from build123d import *

# Parameters (mm, degrees)
ESBO_O1_W                = 22
ESBO_O1_H                = 36
RESSALTO_EXTRUS_O1_DEPTH = 250
CASCA1_T                 = -2
ESBO_O2_R                = 5
CORTE_EXTRUS_O1_DEPTH    = 10
ESBO_O3_R                = 2.75
CORTE_EXTRUS_O2_DEPTH    = 29


with BuildPart() as part:
    # Esboço1 → Ressalto-extrusão1 (new body)
    with BuildSketch(Plane.XY):
        with Locations((0, 18)):
            Rectangle(ESBO_O1_W, ESBO_O1_H)
    extrude(amount=RESSALTO_EXTRUS_O1_DEPTH)

    # Casca1
    casca1_openings = [part.faces().sort_by_distance(p)[0] for p in [
        (0, 18, 0),
    ]]
    offset(amount=CASCA1_T, openings=casca1_openings, kind=Kind.INTERSECTION)

    # Esboço2 → Corte-extrusão1 (cut)
    with BuildSketch(Plane(origin=(0, 0, 0), x_dir=(-1, 0, 0), z_dir=(0, -1, 0))):
        with Locations(Location((0, -20, 0), (0, 0, 90))):
            Circle(ESBO_O2_R)
        with Locations(Location((0, -40, 0), (0, 0, 90))):
            Circle(ESBO_O2_R)
        with Locations(Location((0, -60, 0), (0, 0, 90))):
            Circle(ESBO_O2_R)
        with Locations(Location((0, -80, 0), (0, 0, 90))):
            Circle(ESBO_O2_R)
        with Locations(Location((0, -100, 0), (0, 0, 90))):
            Circle(ESBO_O2_R)
    extrude(amount=-CORTE_EXTRUS_O1_DEPTH, mode=Mode.SUBTRACT)

    # Esboço3 → Corte-extrusão2 (cut)
    with BuildSketch(Plane(origin=(11, 0, 0), x_dir=(0, 0, -1), z_dir=(1, 0, 0))):
        with Locations(Location((-230, 18, 0), (0, 0, 90))):
            Circle(ESBO_O3_R)
    extrude(amount=-CORTE_EXTRUS_O2_DEPTH, mode=Mode.SUBTRACT)


solid = part.part
Here's how the part is built. I have some questions about the finished solid (model axes, mm). A direction names the side the tool comes from. Coordinates: 2 decimals unless noted, no trailing zeros. Order: outer loops, then holes, each group sorted by start corner. A loop starts at its lowest first (then second) coordinate and runs counter-clockwise, first axis right, second up. Notation, with made-up numbers: (83.5, 49) - (123.5, 49) arc R20 ccw to (123.5, 63) - close; hole circle Ø10 at (-9, 89). An arc over 180 degrees is marked (long way). Use CSV: the item, a comma, the result in double quotes. Start each with the question number.
1. Suppose I cut it at A-A on z = 230. List the corners of the cut face in (x, y) for me, then the cut area to 3 significant figures.
2. For faces 5 (the face through (0, 1, 65)), 6 (the face through (0, 2, 122)), 7 (the face through (10.014, 17.404, 227.315)), which set-ups out of +Z, -Z, +X, -X, +Y, -Y let a thin tool reach every point of the face, with its end or its side?
3. Please list where these lines run through material, in increasing order: line 1 (X direction, y = 17.5, z = 140.5); line 2 (Z direction, x = -9.7, y = 18); line 3 (X direction, y = 0.6, z = 100). Write a range as from..to.
4. I'm going to push flat-ended pins straight in: pin 1 (9 mm diameter, centred on x = 0, z = 80, fed in from -Y); pin 2 (1 mm diameter, centred on x = -4, y = 26.5, fed in from -Z). Where does each tip first touch, or does it pass through?
5. Suppose I cut it at C-C on z = 116.5. List the corners of the cut face in (x, y) for me.
6. Suppose I cut it at B-B on y = 18. List the corners of the cut face in (x, z) for me.
7. If we mould it in two halves opening along Y, with no side actions, what happens to faces 1 (the face through (0, 36, 123)), 2 (the face through (0, 34, 122)), 3 (the face through (0, 18, 248)), 4 (the face through (-1.915, 0.986, 75.381))? For each: +Y half, -Y half, draft (parallel to the pull), parting line (faces both ways), or undercut.
8. Suppose I cut it at D-D on x = 0. List the corners of the cut face in (y, z) for me, then the cut area to 3 significant figures.
Output:
1,outline,"(-11, 0) - (11, 0) - (11, 15.25) - (9, 15.25) - (9, 2) - (-9, 2) - (-9, 15.25) - (-11, 15.25) - close; (-11, 20.75) - (-9, 20.75) - (-9, 34) - (9, 34) - (9, 20.75) - (11, 20.75) - (11, 36) - (-11, 36) - close"
1,area,"194 mm2"
2,face 5,"-Y"
2,face 6,"-Z"
2,face 7,"+X, -X"
3,line 1,"x = -11..-9, 9..11"
3,line 2,"z = 0..227.25, 232.75..250"
3,line 3,"x = -11..-5, 5..11"
4,pin 1,"stops at y = 34"
4,pin 2,"stops at z = 248"
5,outline,"(-11, 0) - (11, 0) - (11, 36) - (-11, 36) - close; hole (-9, 2) - (9, 2) - (9, 34) - (-9, 34) - close"
6,outline,"(-11, 0) - (-9, 0) - (-9, 227.25) - (-11, 227.25) - close; (-11, 232.75) - (-9, 232.75) - (-9, 248) - (9, 248) - (9, 232.75) - (11, 232.75) - (11, 250) - (-11, 250) - close; (9, 0) - (11, 0) - (11, 227.25) - (9, 227.25) - close"
7,face 1,"+Y half"
7,face 2,"undercut"
7,face 3,"undercut"
7,face 4,"draft"
8,outline,"(0, 0) - (2, 0) - (2, 15) - (0, 15) - close; (0, 25) - (2, 25) - (2, 35) - (0, 35) - close; (0, 45) - (2, 45) - (2, 55) - (0, 55) - close; (0, 65) - (2, 65) - (2, 75) - (0, 75) - close; (0, 85) - (2, 85) - (2, 95) - (0, 95) - close; (0, 105) - (2, 105) - (2, 248) - (34, 248) - (34, 0) - (36, 0) - (36, 250) - (0, 250) - close"
8,area,"964 mm2"
